from build123d import *

# Parameters (mm, degrees)
F0_W     = 298.45
F0_H     = 298.45
F0_R     = 98.425
F0_R_2   = 84.455
F1_DEPTH = 12.7
F2_DEPTH = 6.35


with BuildPart() as f1:
    # F0 (on Top) → F1 (new body)
    with BuildSketch(Plane.XY):
        Rectangle(F0_W, F0_H)
        Circle(F0_R, mode=Mode.SUBTRACT)
        Circle(F0_R)
        Circle(F0_R_2, mode=Mode.SUBTRACT)
        Circle(F0_R_2)
    extrude(amount=F1_DEPTH)

    # F0 (on Top) → F2 (cut)
    with BuildSketch(Plane.XY):
        Circle(F0_R)
        Circle(F0_R_2, mode=Mode.SUBTRACT)
    extrude(amount=F2_DEPTH, mode=Mode.SUBTRACT)


solid = f1.part
Verification items for the finished model (mm, model axes). A direction names the side the tool comes from. Round coordinates to 2 decimals unless told otherwise and drop trailing zeros. Order: outer loops, then holes, each group sorted by start corner. A loop starts at its lowest first (then second) coordinate and runs counter-clockwise, first axis right, second up.
1. Release check for a two-part mould opening along Y. For faces 3 (the cylindrical face through (38.971, -74.926, 3.131)), 4 (the flat face through (-2, 2, 12.7)), 5 (the cylindrical face through (93.88, 29.56, 3.13)), 6 (the flat face through (-2, 149.225, 6)) record: +Y half, -Y half, draft (parallel to the pull), parting line (faces both ways), or undercut.
Final values:
face 3: undercut
face 4: draft
face 5: undercut
face 6: +Y half
2. Go/stop test with a flat-tipped pin: P1, Ø12, axis at x = 87.5, y = 32, coming from the -Z side. Record where the tip stops, or that it passes through.
Final values:
P1: stops at z = 0
3. Access from +Z, -Z, +X, -X, +Y, -Y to the whole of each face (thin tool, end or side, straight path). Record for faces 1 (the flat face through (-1, 1, 0)), 2 (the flat face through (43, 73, 6.35)).
Final values:
face 1: -Z, +X, -X, +Y, -Y
face 2: -Z
4. Section check A-A on x = 0. Record the cut outline in (y, z) (3 decimals), then the cut area to 3 significant figures.
Final values:
outline: (-149.225, 0) - (-98.425, 0) - (-98.425, 6.35) - (-84.455, 6.35) - (-84.455, 0) - (84.455, 0) - (84.455, 6.35) - (98.425, 6.35) - (98.425, 0) - (149.225, 0) - (149.225, 12.7) - (-149.225, 12.7) - close
area: 3,610 mm2
5. Thickness scan on L1, parallel to Y at x = 0, z = 5.25 (3 decimals); L2, parallel to X at y = -77, z = 5 (3 decimals); L3, parallel to Y at x = 23, z = 1.75 (3 decimals). Record the ranges inside material, lowest first.
Final values:
L1: y = -149.225 to -98.425, -84.455 to 84.455, 98.425 to 149.225
L2: x = -149.225 to -61.306, -34.694 to 34.694, 61.306 to 149.225
L3: y = -149.225 to -95.7, -81.263 to 81.263, 95.7 to 149.225
